from build123d import *

# Parameters (mm, degrees)
SKETCH2_W           = 141
SKETCH2_H           = 8
SKETCH2_W_2         = 8
SKETCH2_H_2         = 28
BOSS_EXTRUDE1_DEPTH = 150
CUT_EXTRUDE1_REACH  = 38
SKETCH3_R           = 4.5
CUT_EXTRUDE2_REACH  = 151
SKETCH5_R           = 4.5
FILLET1_R           = 5
CUT_EXTRUDE3_REACH  = 10


with BuildPart() as part:
    # Sketch2 → Boss-Extrude1 (new body)
    with BuildSketch(Plane.XY):
        with Locations((70.5, 4)):
            Rectangle(SKETCH2_W, SKETCH2_H)
        with Locations((145, 4)):
            Rectangle(SKETCH2_W_2, SKETCH2_H)
        with Locations((145, 22)):
            Rectangle(SKETCH2_W_2, SKETCH2_H_2)
        with Locations((145, -14)):
            Rectangle(SKETCH2_W_2, SKETCH2_H_2)
    extrude(amount=BOSS_EXTRUDE1_DEPTH)

    # Sketch3 → Cut-Extrude1 (cut, up to next)
    with BuildSketch(Plane.XZ, mode=Mode.PRIVATE) as cut_extrude1_sk1:
        with Locations((96.6, 136)):
            Circle(SKETCH3_R)
    cut_extrude1_tool1 = extrude(cut_extrude1_sk1.sketch, amount=-CUT_EXTRUDE1_REACH, mode=Mode.PRIVATE) & part.part
    add(cut_extrude1_tool1.solids().sort_by_distance((96.6, 0, 136))[0], mode=Mode.SUBTRACT)
    # Sketch3 → Cut-Extrude1 (cut, up to next)
    with BuildSketch(Plane.XZ, mode=Mode.PRIVATE) as cut_extrude1_sk2:
        with Locations((16.6, 136)):
            Circle(SKETCH3_R)
    cut_extrude1_tool2 = extrude(cut_extrude1_sk2.sketch, amount=-CUT_EXTRUDE1_REACH, mode=Mode.PRIVATE) & part.part
    add(cut_extrude1_tool2.solids().sort_by_distance((16.6, 0, 136))[0], mode=Mode.SUBTRACT)
    # Sketch3 → Cut-Extrude1 (cut, up to next)
    with BuildSketch(Plane.XZ, mode=Mode.PRIVATE) as cut_extrude1_sk3:
        with Locations((16.6, 14)):
            Circle(SKETCH3_R)
    cut_extrude1_tool3 = extrude(cut_extrude1_sk3.sketch, amount=-CUT_EXTRUDE1_REACH, mode=Mode.PRIVATE) & part.part
    add(cut_extrude1_tool3.solids().sort_by_distance((16.6, 0, 14))[0], mode=Mode.SUBTRACT)
    # Sketch3 → Cut-Extrude1 (cut, up to next)
    with BuildSketch(Plane.XZ, mode=Mode.PRIVATE) as cut_extrude1_sk4:
        with Locations((96.6, 14)):
            Circle(SKETCH3_R)
    cut_extrude1_tool4 = extrude(cut_extrude1_sk4.sketch, amount=-CUT_EXTRUDE1_REACH, mode=Mode.PRIVATE) & part.part
    add(cut_extrude1_tool4.solids().sort_by_distance((96.6, 0, 14))[0], mode=Mode.SUBTRACT)

    # Sketch5 → Cut-Extrude2 (cut, up to next)
    with BuildSketch(Plane(origin=(149, 0, 0), x_dir=(0, 0, -1), z_dir=(1, 0, 0)), mode=Mode.PRIVATE) as cut_extrude2_sk1:
        with Locations((-125, 24)):
            Circle(SKETCH5_R)
    cut_extrude2_tool1 = extrude(cut_extrude2_sk1.sketch, amount=-CUT_EXTRUDE2_REACH, mode=Mode.PRIVATE) & part.part
    add(cut_extrude2_tool1.solids().sort_by_distance((149, 24, 125))[0], mode=Mode.SUBTRACT)
    # Sketch5 → Cut-Extrude2 (cut, up to next)
    with BuildSketch(Plane(origin=(149, 0, 0), x_dir=(0, 0, -1), z_dir=(1, 0, 0)), mode=Mode.PRIVATE) as cut_extrude2_sk2:
        with Locations((-25, 24)):
            Circle(SKETCH5_R)
    cut_extrude2_tool2 = extrude(cut_extrude2_sk2.sketch, amount=-CUT_EXTRUDE2_REACH, mode=Mode.PRIVATE) & part.part
    add(cut_extrude2_tool2.solids().sort_by_distance((149, 24, 25))[0], mode=Mode.SUBTRACT)
    # Sketch5 → Cut-Extrude2 (cut, up to next)
    with BuildSketch(Plane(origin=(149, 0, 0), x_dir=(0, 0, -1), z_dir=(1, 0, 0)), mode=Mode.PRIVATE) as cut_extrude2_sk3:
        with Locations((-25, -16)):
            Circle(SKETCH5_R)
    cut_extrude2_tool3 = extrude(cut_extrude2_sk3.sketch, amount=-CUT_EXTRUDE2_REACH, mode=Mode.PRIVATE) & part.part
    add(cut_extrude2_tool3.solids().sort_by_distance((149, -16, 25))[0], mode=Mode.SUBTRACT)
    # Sketch5 → Cut-Extrude2 (cut, up to next)
    with BuildSketch(Plane(origin=(149, 0, 0), x_dir=(0, 0, -1), z_dir=(1, 0, 0)), mode=Mode.PRIVATE) as cut_extrude2_sk4:
        with Locations((-125, -16)):
            Circle(SKETCH5_R)
    cut_extrude2_tool4 = extrude(cut_extrude2_sk4.sketch, amount=-CUT_EXTRUDE2_REACH, mode=Mode.PRIVATE) & part.part
    add(cut_extrude2_tool4.solids().sort_by_distance((149, -16, 125))[0], mode=Mode.SUBTRACT)

    # Fillet1
    fillet1_edges = [part.edges().sort_by_distance(p)[0] for p in [
        (141, 8, 75),
        (141, 0, 75),
    ]]
    fillet(fillet1_edges, radius=FILLET1_R)

    # Sketch6 → Cut-Extrude3 (cut, up to next)
    with BuildSketch(Plane.ZY.offset(-141), mode=Mode.PRIVATE) as cut_extrude3_sk1:
        with BuildLine():
            Line((50, -5), (100, -5))
            add(Edge.make_bspline(
                [(124, -28), (117.235743552, -28), (112, -16.5), (106.764256448, -5), (100, -5)],
                knots=[0, 0, 0, 0, 0.5, 1, 1, 1, 1], degree=3))
            Line((124, -28), (26, -28))
            add(Edge.make_bspline(
                [(26, -28), (32.764256448, -28), (38, -16.5), (43.235743552, -5), (50, -5)],
                knots=[0, 0, 0, 0, 0.5, 1, 1, 1, 1], degree=3))
        make_face()
    cut_extrude3_tool1 = extrude(cut_extrude3_sk1.sketch, amount=-CUT_EXTRUDE3_REACH, mode=Mode.PRIVATE) & part.part
    add(cut_extrude3_tool1.solids().sort_by_distance((141, -17.262694, 75))[0], mode=Mode.SUBTRACT)


solid = part.part
Model file for the job. Use its own axes, mm. A direction names the side the tool comes from. Round coordinates to 2 decimals unless told otherwise and drop trailing zeros. Order: outer loops, then holes, each group sorted by start corner. A loop starts at its lowest first (then second) coordinate and runs counter-clockwise, first axis right, second up.
(1) Band-saw the part on C-C (y = 24). List the corners of the cut face in (x, z), then the cut area to 3 significant figures.
(2) Pull direction Z, two halves, no side cores. Call faces 1 (the face through (91, 7, 0)), 2 (the face through (141, 24, 74)), 3 (the face through (145.06, 27.04, 28.32)), 4 (the face through (91, 7, 150)): released by +Z, released by -Z, zero draft, split by the parting line, or undercut.
(3) Drill centre lines: line 1 (Z direction, x = 16, y = 4); line 2 (Y direction, x = 146, z = 25); line 3 (Y direction, x = 19, z = 92.5). Where is each one in solid material? Low to high.
(4) 3-axis set-ups, long thin cutter, end or side, ignore diameter. For faces 5 (the face through (145, -5, 75)), 6 (the face through (15.62, 3.94, 131.61)), 7 (the face through (145, 36, 74)), 8 (the face through (141, -17, 130)), 9 (the face through (69, 8, 74)): which of +Z, -Z, +X, -X, +Y, -Y reach the whole face in a straight line?
(5) Band-saw the part on A-A (z = 14). List the corners of the cut face in (x, y), then the cut area to 3 significant figures.
(6) Band-saw the part on B-B (x = 16.6). List the corners of the cut face in (y, z).
(7) Pin check, flat tips, straight feed: pin 1 (10.5 mm diameter, centred on x = 96.6, z = 136, fed in from -Y); pin 2 (8 mm diameter, centred on x = 16.6, z = 14, fed in from -Y); pin 3 (14.5 mm diameter, centred on x = 16.6, z = 136, fed in from +Y); pin 4 (14.5 mm diameter, centred on y = -16, z = 125, fed in from -X). Stop position of each tip, or through.
(8) Band-saw the part on D-D (z = 53). List the corners of the cut face in (x, y).
Verdict:
1. outline: (141, 0) - (149, 0) - (149, 20.5) - (141, 20.5) - close; (141, 29.5) - (149, 29.5) - (149, 120.5) - (141, 120.5) - close; (141, 129.5) - (149, 129.5) - (149, 150) - (141, 150) - close
1. area: 1,060 mm2
2. face 1: released by -Z
2. face 2: zero draft
2. face 3: undercut
2. face 4: released by +Z
3. line 1: z = 0 to 9.54, 18.46 to 131.54, 140.46 to 150
3. line 2: y = -28 to -20.5, -11.5 to 19.5, 28.5 to 36
3. line 3: y = 0 to 8
4. face 5: +X, -X, -Y
4. face 6: +Y, -Y
4. face 7: +Z, -Z, +X, -X, +Y
4. face 8: +Z, -Z, -X, -Y
4. face 9: +Z, -Z, -X, +Y
5. outline: (0, 0) - (12.1, 0) - (12.1, 8) - (0, 8) - close; (21.1, 0) - (92.1, 0) - (92.1, 8) - (21.1, 8) - close; (101.1, 0) - (136, 0) arc R5 cw to (141, -5) - (141, -28) - (149, -28) - (149, 36) - (141, 36) - (141, 13) arc R5 cw to (136, 8) - (101.1, 8) - close
5. area: 1,510 mm2
6. outline: (0, 0) - (8, 0) - (8, 9.5) - (0, 9.5) - close; (0, 18.5) - (8, 18.5) - (8, 131.5) - (0, 131.5) - close; (0, 140.5) - (8, 140.5) - (8, 150) - (0, 150) - close
7. pin 1: stops at y = 0
7. pin 2: passes through
7. pin 3: stops at y = 8
7. pin 4: stops at x = 141
8. outline: (0, 0) - (136, 0) arc R5 cw to (141, -5) - (149, -5) - (149, 36) - (141, 36) - (141, 13) arc R5 cw to (136, 8) - (0, 8) - close
